from build123d import *

# Parameters (mm, degrees)
SKETCH1_W           = 190
SKETCH1_H           = 50
SKETCH1_R           = 15
SKETCH1_R_2         = 1.5
SKETCH1_R_3         = 3
BOSS_EXTRUDE1_DEPTH = 5
CUT_EXTRUDE1_START  = -5
SKETCH2_R           = 2.75
CUT_EXTRUDE1_DEPTH  = 1.5


with BuildPart() as part:
    # Sketch1 → Boss-Extrude1 (new body)
    with BuildSketch(Plane.XY):
        with Locations((95, 25)):
            Rectangle(SKETCH1_W, SKETCH1_H)
        with Locations((25, 25)):
            Circle(SKETCH1_R, mode=Mode.SUBTRACT)
        with Locations((165, 25)):
            Circle(SKETCH1_R, mode=Mode.SUBTRACT)
        with Locations((35, 7)):
            Circle(SKETCH1_R_2, mode=Mode.SUBTRACT)
        with Locations((175, 7)):
            Circle(SKETCH1_R_2, mode=Mode.SUBTRACT)
        with Locations((155, 7)):
            Circle(SKETCH1_R_2, mode=Mode.SUBTRACT)
        with Locations((70.5, 20)):
            Circle(SKETCH1_R_2, mode=Mode.SUBTRACT)
        with Locations((86, 7.5)):
            Circle(SKETCH1_R_3, mode=Mode.SUBTRACT)
        with Locations((104, 7.5)):
            Circle(SKETCH1_R_3, mode=Mode.SUBTRACT)
        with Locations((15, 7)):
            Circle(SKETCH1_R_2, mode=Mode.SUBTRACT)
        with Locations((52.5, 4)):
            Circle(SKETCH1_R_2, mode=Mode.SUBTRACT)
        with Locations((52.5, 20)):
            Circle(SKETCH1_R_2, mode=Mode.SUBTRACT)
        with Locations((70.5, 4)):
            Circle(SKETCH1_R_2, mode=Mode.SUBTRACT)
    extrude(amount=BOSS_EXTRUDE1_DEPTH)

    # Sketch2 → Cut-Extrude1 (cut)
    with BuildSketch(Plane.XY.offset(5).offset(CUT_EXTRUDE1_START)):
        with Locations((15, 7)):
            Circle(SKETCH2_R)
        with Locations((35, 7)):
            Circle(SKETCH2_R)
        with Locations((155, 7)):
            Circle(SKETCH2_R)
        with Locations((175, 7)):
            Circle(SKETCH2_R)
    extrude(amount=CUT_EXTRUDE1_DEPTH, mode=Mode.SUBTRACT)


solid = part.part
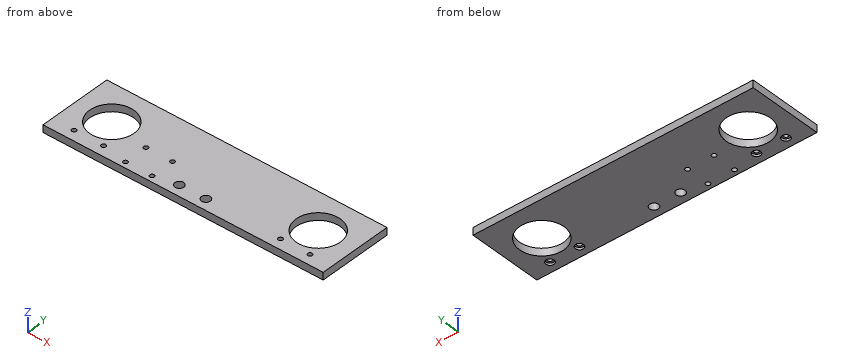
Geometry check sheet. Reference: the model listing, model coordinates, mm. Give positions to 0.01 mm unless a question says otherwise; leave off trailing zeros. Write each loop counter-clockwise with the first axis right and the second up, starting at its lowest first coordinate (ties: lowest second). Pieces come first, ordered by that corner, then holes. Notation, with made-up numbers: M 60.25,-6 L 79.25,-6 A27 ccw 79.25,20 Z; hole C -28.5,-10 d9. An arc over 180 degrees is marked long. Answer as CSV lines item,"result". Start each with the question number.
Q1. Section check A-A, the plane z = 3.9. Give the number of separate pieces and of enclosed holes in the cut face, then the cut area to 3 significant figures.
Q2. Section check C-C, the plane y = 37.5. Record the cut outline in (x, z), then the cut area to 3 significant figures.
Q3. Section check D-D, the plane x = 25. Record the cut outline in (y, z), then the cut area to 3 significant figures.
Q4. Material ranges on L1, parallel to X at y = 9.5, z = 2.45; L2, parallel to Y at x = 154, z = 2.4; L3, parallel to X at y = 12.5, z = 2.35, recorded low to high.
Q5. Section check B-B, the plane x = 104. Record the cut outline in (y, z).
Q6. Go/stop test with flat-tipped pins: pin 1 (1.8 mm diameter, centred on x = 52.5, y = 20, fed in from -Z); pin 2 (1.6 mm diameter, centred on x = 36, y = 6, fed in from -Z). Record where each tip stops, or that it passes through.
Geometry says:
1,separate pieces,"1"
1,enclosed holes,"12"
1,area,"7,970 mm^2"
2,outline,"M 0,0 L 16.71,0 L 16.71,5 L 0,5 Z; M 33.29,0 L 156.71,0 L 156.71,5 L 33.29,5 Z; M 173.29,0 L 190,0 L 190,5 L 173.29,5 Z"
2,area,"784 mm^2"
3,outline,"M 0,0 L 10,0 L 10,5 L 0,5 Z; M 40,0 L 50,0 L 50,5 L 40,5 Z"
3,area,"100 mm^2"
4,L1,"0 to 83.76, 88.24 to 101.76, 106.24 to 190"
4,L2,"0 to 5.88, 8.12 to 14.8, 35.2 to 50"
4,L3,"0 to 16.71, 33.29 to 156.71, 173.29 to 190"
5,outline,"M 0,0 L 4.5,0 L 4.5,5 L 0,5 Z; M 10.5,0 L 50,0 L 50,5 L 10.5,5 Z"
6,pin 1,"through"
6,pin 2,"z = 1.5"
